Build history of the part. All positions in model axes, mm. A direction names the side the tool comes from. Round coordinates to 2 decimals unless told otherwise and drop trailing zeros. Loops run counter-clockwise (first coordinate to the right, second up) from the corner with the lowest first, then second, coordinate; pieces in that order, holes last. Notation, with made-up numbers: M -20,54.5 L 15,54.5 A20 cw 15,75.5 Z; hole C 44,44.25 d1. An arc over 180 degrees is marked long. One line per item, written item: value.
```python
from build123d import *

# Parameters (mm, degrees)
F0_W     = 270
F0_H     = 150
F1_DEPTH = 250
F2_R     = 80
F3_T     = -2.5
F5_DEPTH = 2.5
F7_DEPTH = 25


with BuildPart() as f1:
    # F0 (on Front) → F1 (new body)
    with BuildSketch(Plane.XZ):
        with Locations((0, 75)):
            Rectangle(F0_W, F0_H)
    extrude(amount=F1_DEPTH)

    # F2
    f2_edges = [f1.edges().sort_by_distance(p)[0] for p in [
        (-135, -125, 150),
        (135, -125, 150),
    ]]
    fillet(f2_edges, radius=F2_R)

    # F3
    f3_openings = [f1.faces().sort_by_distance(p)[0] for p in [
        (0, -125, 0),
    ]]
    offset(amount=F3_T, openings=f3_openings)

    # F4 (on face) → F5 (cut, through all)
    with BuildSketch(Plane.XZ.offset(250)):
        with BuildLine():
            Line((-15, 60), (-15, 0))
            Line((-15, 0), (65, 0))
            Line((65, 0), (65, 60))
            ThreePointArc((65, 60), (56.213203, 81.213203), (35, 90))
            Line((35, 90), (15, 90))
            ThreePointArc((15, 90), (-6.213203, 81.213203), (-15, 60))
        make_face()
    extrude(amount=-F5_DEPTH, mode=Mode.SUBTRACT)

    # F6 (on face) → F7 (cut)
    with BuildSketch(Plane(origin=(0, 0, 0), x_dir=(-1, 0, 0), z_dir=(0, 1, 0))):
        with BuildLine():
            Line((25, 60), (25, 0))
            Line((25, 0), (105, 0))
            Line((105, 0), (105, 60))
            ThreePointArc((105, 60), (96.213203, 81.213203), (75, 90))
            Line((75, 90), (55, 90))
            ThreePointArc((55, 90), (33.786797, 81.213203), (25, 60))
        make_face()
    extrude(amount=-F7_DEPTH, mode=Mode.SUBTRACT)


solid = f1.part
```
Item 1: Slice it at D-D, the plane z = 105. Give the cut face in (x, y).
Check values:
outline: M -126.94,-250 L 126.94,-250 L 126.94,0 L -126.94,0 Z; hole M -124.15,-247.5 L 124.15,-247.5 L 124.15,-2.5 L -124.15,-2.5 Z
Item 2: Slice it at A-A, the plane z = 23. Give the cut face in (x, y).
Check values:
outline: M -135,-250 L -15,-250 L -15,-247.5 L -132.5,-247.5 L -132.5,-2.5 L -105,-2.5 L -105,0 L -135,0 Z; M -25,-2.5 L 132.5,-2.5 L 132.5,-247.5 L 65,-247.5 L 65,-250 L 135,-250 L 135,0 L -25,0 Z
Item 3: Slice it at C-C, the plane x = 68.5. Give the cut face in (y, z), and give its area (3 significant figures).
Check values:
outline: M -250,0 L -247.5,0 L -247.5,146.32 L -2.5,146.32 L -2.5,0 L 0,0 L 0,148.85 L -250,148.85 Z
area: 1,370 mm2
Item 4: Which spindle directions (+Z, -Z, +X, -X, +Y, -Y) get a long thin tool onto all of the face, cutting with end or side? Do faces 1 (the face through (-34.021, -1.232, 81.445)), 2 (the face through (56.445, -248.768, 80.979)), 3 (the face through (110.4, -126.715, 124.195)), 4 (the face through (-2, -250, 93)), 5 (the face through (-133, -124, 0)). Say none if no direction does.
Check values:
face 1: -Z, +Y
face 2: -Z, -Y
face 3: -Z
face 4: +Z, -Z, +X, -X, -Y
face 5: -Z, +X, -X, +Y, -Y
Item 5: Drop flat-ended pins along their axis: P1, Ø2, axis at x = 24.5, y = -248.5, coming from the -Z side; P2, Ø8, axis at x = -45.5, y = -166, coming from the -Z side; P3, Ø12, axis at y = -220, z = 103.5, coming from the +X side. Give the stop position or say it passes through.
Check values:
P1: stops at z = 90
P2: stops at z = 147.5
P3: stops at x = 130.12
Item 6: Wall check: line 1 along X through (y, z) = (-162, 8); line 2 along Y through (x, z) = (92, 88); line 3 along Z through (x, y) = (-15.5, -36.5). Give the ranges that are in metal, low to high.
Check values:
line 1: x = -135 to -132.5, 132.5 to 135
line 2: y = -250 to -247.5, -2.5 to 0
line 3: z = 147.5 to 150
Item 7: Pull direction X, two halves, no side cores. Call faces 6 (the face through (-1, -123, 147.5)), 7 (the face through (-135, -123, 35)), 8 (the face through (-132.5, -123, 35)), 9 (the face through (112.19, -126.75, 125.94)): pulls with the +X half, pulls with the -X half, needs draft (parallel to the pull), parting line crosses it, or undercut.
Check values:
face 6: undercut
face 7: pulls with the -X half
face 8: undercut
face 9: pulls with the +X half
Item 8: Slice it at B-B, the plane y = -102. Give the cut face in (x, z).
Check values:
outline: M -135,0 L -132.5,0 L -132.5,70 A77.5 cw -55,147.5 L 55,147.5 A77.5 cw 132.5,70 L 132.5,0 L 135,0 L 135,70 A80 ccw 55,150 L -55,150 A80 ccw -135,70 Z
